Build history of the part. All positions in model axes, mm. Face numbers are marked on the shaded views. A direction names the side the tool comes from. Coordinates: 2 decimals unless noted, no trailing zeros. Loops run counter-clockwise (first coordinate to the right, second up) from the corner with the lowest first, then second, coordinate; pieces in that order, holes last. Notation, with made-up numbers: (-29, 55) -> (-9, 55) arc R22 cw to (-9, 87) -> close; hole circle Ø7 at (62, 68). An arc over 180 degrees is marked (long way). One line per item, written item: value. Start each with the question number.
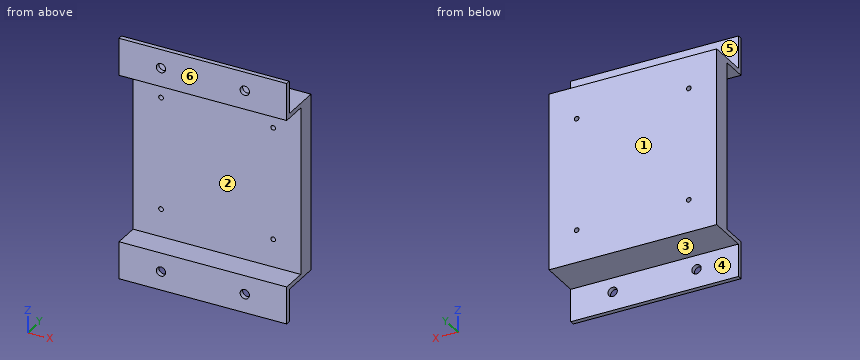
Autodesk Inventor part; units mm, degrees
ref_plane "YZ Plane" through (0, 0, 0) normal (1, 0, 0) x (0, 1, 0)
ref_plane "XZ Plane" through (0, 0, 0) normal (0, 1, 0) x (-1, 0, 0)
ref_plane "XY Plane" through (0, 0, 0) normal (0, 0, 1) x (1, 0, 0)
sketch "Sketch1" plane through (0, 0, 0) normal (0, 1, 0) x (-1, 0, 0)
  line L0 (0, 0) -> (-114.3, 0)
  line L1 (-114.3, 0) -> (-114.3, -114.3)
  line L2 (-114.3, -114.3) -> (0, -114.3)
  line L3 (0, -114.3) -> (0, 0)
  dimension "d0" = 114.3
  dimension "d1" = 114.3
extrude "Extrusion1" add sketch "Sketch1" along normal blind 3.175
sketch "Sketch2" plane through (0, 0, 0) normal (0, 0, 1) x (1, 0, 0)
  line L0 (114.3, 3.175) -> (0, 3.175)
  line L1 (0, 3.175) -> (114.3, 3.175)
  line L2 (0, 0) -> (0, 3.175)
  line L3 (0, 3.175) -> (114.3, 3.175)
  line L4 (114.3, 3.175) -> (114.3, -26.9875)
  line L5 (114.3, -26.9875) -> (0, -26.9875)
  line L6 (0, -26.9875) -> (0, 3.175)
  dimension "d14" = 30.1625
extrude "Extrusion2" add sketch "Sketch2" along normal blind 3.175
sketch "Sketch5" plane through (114.3, 0, -114.3) normal (0, 0, -1) x (-1, 0, 0)
  line L0 (114.3, 3.175) -> (114.3, -26.9875)
  line L1 (0, 3.175) -> (114.3, 3.175)
  line L2 (114.3, 3.175) -> (114.3, -26.9875)
  line L3 (114.3, -26.9875) -> (0, -26.9875)
  line L4 (0, -26.9875) -> (0, 3.175)
  point P0 (114.3, 0)
extrude "Extrusion5" add sketch "Sketch5" along normal blind 3.175
sketch "Sketch6" plane through (0, -26.9875, -114.3) normal (0, -1, 0) x (1, 0, 0)
  line L0 (114.3, 114.3) -> (114.3, 0)
  line L1 (114.3, 0) -> (0, 0)
  line L2 (0, 0) -> (0, -25.4)
  line L3 (0, -25.4) -> (114.3, -25.4)
  line L4 (114.3, -25.4) -> (114.3, 0)
  line L5 (0, 114.3) -> (114.3, 114.3)
  line L6 (114.3, 114.3) -> (0, 114.3)
  line L7 (0, 114.3) -> (0, 139.7)
  line L8 (0, 139.7) -> (114.3, 139.7)
  line L9 (114.3, 139.7) -> (114.3, 114.3)
  dimension "d17" = 25.4
  dimension "d18" = 25.4
extrude "Extrusion6" add sketch "Sketch6" against normal blind 3.175
sketch "Sketch7" plane through (0, -23.8125, -114.3) normal (0, 1, 0) x (1, 0, 0)
  point P0 (0, -114.3)
sketch "Sketch8" plane through (0, 3.175, 0) normal (0, 1, 0) x (1, 0, 0)
  circle A0 centre (19.0626, 18.7934) radius 1.5875
  circle A1 centre (19.0626, 95.3281) radius 1.5875
  circle A2 centre (95.4804, 18.7934) radius 1.5875
  circle A3 centre (95.4804, 95.3281) radius 1.5875
  point P0 (0, 0)
  dimension "d21" = 3.175
  dimension "d22" = 3.175
  dimension "d23" = 3.175
  dimension "d24" = 3.175
extrude "Extrusion7" cut sketch "Sketch8" against normal blind 12.7
sketch "Sketch9" plane through (0, -23.8125, -114.3) normal (0, 1, 0) x (1, 0, 0)
  line L0 (114.3, -139.7) -> (0, -139.7) construction
  line L1 (0, -139.7) -> (0, -127) construction
  line L2 (0, -114.3) -> (0, -139.7) construction
  line L3 (0, -139.7) -> (12.7, -139.7) construction
  line L4 (114.3, -114.3) -> (114.3, -139.7) construction
  line L5 (0, -127) -> (28.575, -127) construction
  line L6 (0, -127) -> (28.575, -127) construction
  line L7 (28.575, -127) -> (85.725, -127) construction
  circle A0 centre (28.575, -127) radius 3.175
  circle A1 centre (85.725, -127) radius 3.175
  line L8 (114.3, 25.4) -> (0, 25.4) construction
  line L9 (0, 25.4) -> (0, 12.7) construction
  line L10 (0, 12.7) -> (28.575, 12.7) construction
  line L11 (28.575, 12.7) -> (85.725, 12.7) construction
  line L12 (28.575, 12.7) -> (85.725, 12.7) construction
  circle A2 centre (28.575, 12.7) radius 3.175
  circle A3 centre (85.725, 12.7) radius 3.175
  dimension "d27" = 12.7
  dimension "d28" = 90
  dimension "d29" = 28.575
  dimension "d30" = 0
  dimension "d31" = 57.15
  dimension "d33" = 6.35
  dimension "d34" = 6.35
  dimension "d35" = 12.7
  dimension "d36" = 28.575
  dimension "d37" = 57.15
  dimension "d39" = 6.35
  dimension "d40" = 6.35
extrude "Extrusion8" cut sketch "Sketch9" against normal blind 3.175
sketch "Sketch10" plane through (0, 0, 0) normal (0, -1, 0) x (1, 0, 0)
  line L0 (0, 0) -> (114.3, 0)
  line L1 (114.3, -117.475) -> (0, -117.475)
  line L2 (114.3, 0) -> (0, 0)
  line L3 (0, 0) -> (0, -117.475)
  line L4 (0, -117.475) -> (114.3, -117.475)
  line L5 (114.3, -117.475) -> (114.3, 0)
  circle A0 centre (95.4804, -18.7934) radius 1.5875
  circle A1 centre (95.4804, -18.7934) radius 1.5875
  circle A2 centre (95.4804, -95.3281) radius 1.5875
  circle A3 centre (95.4804, -95.3281) radius 1.5875
  circle A4 centre (19.0626, -18.7934) radius 1.5875
  circle A5 centre (19.0626, -18.7934) radius 1.5875
  circle A6 centre (19.0626, -95.3281) radius 1.5875
  circle A7 centre (19.0626, -95.3281) radius 1.5875
  dimension "d45" = 3.175
  dimension "d46" = 3.175
  dimension "d47" = 3.175
  dimension "d48" = 3.175
extrude "Extrusion9" add sketch "Sketch10" along normal blind 9.525
properties part number "TurntableBase"
Item 1: Band-saw the part on C-C, the plane x = 11. List the corners of the cut face in (y, z) (1 decimal).
Item 2: Two-plate mould, pull along Z, no slides. Class the marked faces 1, 2 and 3: +Z half, -Z half, draft (parallel to the pull), parting line (faces both ways), or undercut.
Item 3: Band-saw the part on D-D, the plane z = -62. List the corners of the cut face in (x, y) (3 decimals).
Item 4: Tool access for the marked faces 4, 5 and 6: list every direction of +Z, -Z, +X, -X, +Y, -Y with a clear straight run to the whole face (end or side of a thin tool).
Item 5: Band-saw the part on A-A, the plane y = -13.5. List the corners of the cut face in (x, z) (3 decimals).
Item 6: Probe probe 1 along X at (y, z) = (-24.55, 12.7); probe 2 along Z at (x, y) = (80, -13.5) (3 decimals); probe 3 along Y at (x, z) = (15, -45) (3 decimals). List the from-to ranges inside material, lowest first.
Item 7: Band-saw the part on B-B, the plane z = 12.7. List the corners of the cut face in (x, y), and give its area (3 significant figures).
Item 8: Drop flat-ended pins along their axis: pin 1 Ø7.5 at (x, z) = (85.725, 12.7) entering from +Y; pin 2 Ø6 at (x, y) = (65, -4.5) entering from +Z (3 decimals); pin 3 Ø4 at (x, z) = (28.575, 12.7) entering from -Y; pin 4 Ø3 at (x, y) = (15.5, -21.5) entering from -Z (3 decimals). Give the stop position or say it passes through.
Worked out:
1. outline: (-27, -139.7) -> (-23.8, -139.7) -> (-23.8, -117.5) -> (3.2, -117.5) -> (3.2, 3.2) -> (-23.8, 3.2) -> (-23.8, 25.4) -> (-27, 25.4) -> (-27, 0) -> (-9.5, 0) -> (-9.5, -114.3) -> (-27, -114.3) -> close
2. face 1: draft
2. face 2: undercut
2. face 3: -Z half
3. outline: (0, -9.525) -> (114.3, -9.525) -> (114.3, 3.175) -> (0, 3.175) -> close
4. face 4: -Z, +X, -X, +Y
4. face 5: +Z, +X, -X, +Y
4. face 6: +Z, -Z, +X, -X, -Y
5. outline: (0, -117.475) -> (114.3, -117.475) -> (114.3, -114.3) -> (0, -114.3) -> close; (0, 0) -> (114.3, 0) -> (114.3, 3.175) -> (0, 3.175) -> close
6. probe 1: x = 0 to 25.4, 31.75 to 82.55, 88.9 to 114.3
6. probe 2: z = -117.475 to -114.3, 0 to 3.175
6. probe 3: y = -9.525 to 3.175
7. outline: (0, -26.99) -> (25.4, -26.99) -> (25.4, -23.81) -> (0, -23.81) -> close; (31.75, -26.99) -> (82.55, -26.99) -> (82.55, -23.81) -> (31.75, -23.81) -> close; (88.9, -26.99) -> (114.3, -26.99) -> (114.3, -23.81) -> (88.9, -23.81) -> close
7. area: 323 mm²
8. pin 1: stops at y = -23.81
8. pin 2: stops at z = 3.175
8. pin 3: passes through
8. pin 4: stops at z = -117.475
